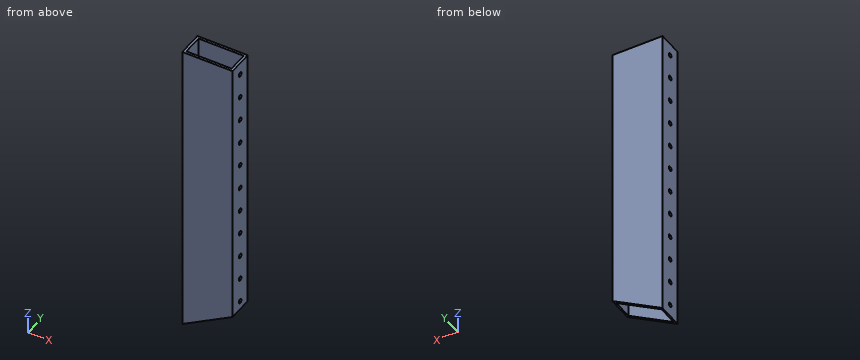
from build123d import *

# Parameters (mm, degrees)
SKETCH1_W             = 50.8
SKETCH1_H             = 25.4
SKETCH1_W_2           = 45.72
SKETCH1_H_2           = 20.32
BOSS_EXTRUDE1_DEPTH   = 533.4
F_8_CLEARANCE_HOLE1_D = 4.4958
CUT_EXTRUDE2_DEPTH    = 76.962
CUT_EXTRUDE4_DEPTH    = 40.64


with BuildPart() as part:
    # Sketch1 → Boss-Extrude1 (new body)
    with BuildSketch(Plane.XY):
        Rectangle(SKETCH1_W, SKETCH1_H)
        Rectangle(SKETCH1_W_2, SKETCH1_H_2, mode=Mode.SUBTRACT)
    extrude(amount=-BOSS_EXTRUDE1_DEPTH)

    # #8 Clearance Hole1 (through all)
    with Locations(Plane(origin=(25.4, 0, 0), x_dir=(0, 0, -1), z_dir=(1, 0, 0))):
        with Locations((12.7, 0), (38.1, 0), (63.5, 0), (88.9, 0), (114.3, 0), (139.7, 0), (165.1, 0), (190.5, 0), (215.9, 0), (241.3, 0), (266.7, 0), (292.1, 0), (317.5, 0), (342.9, 0), (368.3, 0), (393.7, 0), (419.1, 0), (444.5, 0), (469.9, 0), (495.3, 0), (520.7, 0)):
            Hole(F_8_CLEARANCE_HOLE1_D / 2)

    # Sketch4 → Cut-Extrude2 (cut)
    with BuildSketch(Plane(origin=(0, 12.7, 0), x_dir=(1, 0, 0), z_dir=(0, 1, 0))):
        Polygon((-7.206301081, 228.6), (135.513081356, 228.6), (135.513081356, -17.641370014), (-94.056886123, -17.641370014), (-94.056886123, 228.6), align=None)
    extrude(amount=-CUT_EXTRUDE2_DEPTH, mode=Mode.SUBTRACT)

    # Sketch6 → Cut-Extrude4 (cut)
    with BuildSketch(Plane(origin=(0, 12.7, 0), x_dir=(1, 0, 0), z_dir=(0, 1, 0))):
        Polygon((-25.4, 533.4), (25.4, 504.070606325), (25.4, 533.4), align=None)
    extrude(amount=-CUT_EXTRUDE4_DEPTH, mode=Mode.SUBTRACT)


solid = part.part
CAD build for the part. Positions are in the model's coordinates, mm. Round coordinates to 2 decimals unless told otherwise and drop trailing zeros. Write each loop counter-clockwise with the first axis right and the second up, starting at its lowest first coordinate (ties: lowest second). Pieces come first, ordered by that corner, then holes. Notation, with made-up numbers: M -32,13 L -25,13 A23 ccw -25,34 Z; hole C -29,22.25 d4. An arc over 180 degrees is marked long. Use a Markdown table: item, result. Add a question column.
1. Slice it at B-B on z = -255. Give the cut face in (x, y), then the cut area to 3 significant figures.
2. Slice it at A-A on y = 6.75. Give the cut face in (x, z).
3. Slice it at C-C on x = -17.5. Give the cut face in (y, z), then the cut area to 3 significant figures.
4. Drill centre lines: probe 1 along X at (y, z) = (8, -502.5); probe 2 along Y at (x, z) = (8, -321); probe 3 along Y at (x, z) = (-23.55, -241.3). Where is each one in solid material? Low to high.
Reply:
| question | item | result |
|---|---|---|
| 1 | outline | M -25.4,-12.7 L 25.4,-12.7 L 25.4,12.7 L -25.4,12.7 Z; hole M -22.86,-10.16 L 22.86,-10.16 L 22.86,10.16 L -22.86,10.16 Z |
| 1 | area | 361 mm^2 |
| 2 | outline | M -25.4,-533.4 L -22.86,-531.93 L -22.86,-228.6 L -25.4,-228.6 Z; M 22.86,-505.54 L 25.4,-504.07 L 25.4,-228.6 L 22.86,-228.6 Z |
| 3 | outline | M -12.7,-528.84 L -10.16,-528.84 L -10.16,-228.6 L -12.7,-228.6 Z; M 10.16,-528.84 L 12.7,-528.84 L 12.7,-228.6 L 10.16,-228.6 Z |
| 3 | area | 1,530 mm^2 |
| 4 | probe 1 | x = -25.4 to -22.86, 22.86 to 25.4 |
| 4 | probe 2 | y = -12.7 to -10.16, 10.16 to 12.7 |
| 4 | probe 3 | y = -12.7 to -2.25, 2.25 to 12.7 |
